For this review, take the finished solid that the model builds, in its own axes (mm). A direction names the side the tool comes from. Round coordinates to 2 decimals unless told otherwise and drop trailing zeros. Write each loop counter-clockwise with the first axis right and the second up, starting at its lowest first coordinate (ties: lowest second). Pieces come first, ordered by that corner, then holes. Notation, with made-up numbers: (65.25, -11.75) -> (88.25, -11.75) arc R24 cw to (88.25, 1.25) -> close; hole circle Ø7 at (3, -40). An arc over 180 degrees is marked (long way). Write item = value, one per line. Start each with the question number.
Autodesk Inventor part; units mm, degrees
ref_plane "Work Plane6" through (0, 0, 176.4284) normal (0, 0, 1) x (1, 0, 0)
ref_plane "Work Plane12" through (0, 0, 148.9464) normal (0, 0, 1) x (1, 0, 0)
ref_plane "Work Plane13" through (0, 0, 49.7586) normal (0, 0, -1) x (-1, 0, 0)
sketch "Sketch1" plane through (0, 0, 0) normal (0, 0, 1) x (1, 0, 0)
  circle A0 centre (0, 0) radius 4.7625
  line L0 (-1.5875, 6.35) -> (1.5875, 6.35)
  line L1 (1.5875, 6.35) -> (1.5875, 3.175)
  line L2 (1.5875, 3.175) -> (-1.5875, 3.175)
  line L3 (-1.5875, 3.175) -> (-1.5875, 6.35)
  dimension "d0" = 9.525
  dimension "d43" = 3.175
  dimension "d44" = 3.175
  dimension "d45" = 1.5875
  dimension "d46" = 6.35
extrude "Extrusion1" add sketch "Sketch1" along normal blind 165.05 contours A0 L3 L2 L1 | L1 L2 L3 A0
ref_plane "Work Plane6" through (0, 0, 176.4284) normal (0, 0, 1) x (1, 0, 0)
ref_plane "Work Plane12" through (0, 0, 148.9464) normal (0, 0, 1) x (1, 0, 0)
sketch "Sketch10" plane through (0, 0, 148.9464) normal (0, 0, 1) x (1, 0, 0)
  circle A0 centre (0, 0) radius 3.8481
  circle A1 centre (0, 0) radius 4.7625
extrude "Extrusion11" cut sketch "Sketch10" along normal blind 1.143
ref_plane "Work Plane13" through (0, 0, 49.7586) normal (0, 0, -1) x (-1, 0, 0)
sketch "Sketch11" plane through (0, 0, 49.7586) normal (0, 0, -1) x (-1, 0, 0)
  circle A0 centre (0, 0) radius 4.7625
  circle A1 centre (0, 0) radius 3.8481
  circle A2 centre (0, 0) radius 4.7625
extrude "Extrusion12" cut sketch "Sketch11" along normal blind 1.143
ref_plane "Work Plane14" through (0, 0, 26.797) normal (0, 0, -1) x (-1, 0, 0)
sketch "Sketch12" plane through (0, 0, 26.797) normal (0, 0, -1) x (-1, 0, 0)
  circle A0 centre (0, 0) radius 3.8481
  circle A1 centre (0, 0) radius 4.7625
extrude "Extrusion13" cut sketch "Sketch12" along normal blind 1.143
ref_plane "Work Plane15" through (0, 0, 148.921) normal (0, 0, 1) x (1, 0, 0)
extrude "Extrusion14" cut sketch "Sketch1" along normal through all contours L1 L2 L3 A0 | A0 L3 L0 L1 picked at (-0.1794, 3.694)
equation "\"d44\" = d43"
properties part number "vertical drive shaft"
1. Clearance check with flat-ended pins moving along their axes: pin 1 Ø1.5 at (x, z) = (2.5, 83) entering from -Y; pin 2 Ø1 at (x, y) = (1.5, -1) entering from -Z; pin 3 Ø0.7 at (y, z) = (4, 76.5) entering from +X; pin 4 Ø0.7 at (y, z) = (4, 57.5) entering from -X. State where each tip first meets the part, or that it passes through.
2. Consider section B-B, the plane z = 145.5. Give the boundary of the cut face in (x, y) (1 decimal).
3. Consider section C-C, the plane y = -2.5. Give the boundary of the cut face in (x, z).
4. Wall thickness on L1, parallel to Z at x = 0.25, y = -4.5; L2, parallel to X at y = 3.5, z = 20; L3, parallel to X at y = 0.5, z = 109: over which ranges is each line inside the solid? List them lowest first. Write a range as from..to.
5. Draft analysis for pull direction Z (two halves, no side actions). For faces 1 (the cylindrical face through (0.19, -4.76, 37.55)), 2 (the flat face through (0, -4, 26.797)), 3 (the flat face through (0, 0, 0)), 4 (the flat face through (0, 0, 165.05)), state which applies: +Z half, -Z half, draft (parallel to the pull), parting line (faces both ways), or undercut.
6. Machinability: for faces 5 (the cylindrical face through (0.19, -4.76, 12.65)), 6 (the cylindrical face through (-0.146, -3.845, 49.195)), 7 (the flat face through (0, 3.175, 81)), which of the approach directions +Z, -Z, +X, -X, +Y, -Y give a long, thin tool a straight path to every point of the face, cutting with its end or side? Answer none if there is none.
Outcome:
q1.pin_1 = -4.43
q1.pin_2 = 0
q1.pin_3 = 3.06
q1.pin_4 = -3.06
q2.outline = (-1.6, 3.2) -> (-1.6, 4.5) arc R4.8 ccw (long way) to (1.6, 4.5) -> (1.6, 3.2) -> close
q3.outline = (-4.05, 0) -> (4.05, 0) -> (4.05, 25.65) -> (2.93, 25.65) -> (2.93, 26.8) -> (4.05, 26.8) -> (4.05, 48.62) -> (2.93, 48.62) -> (2.93, 49.76) -> (4.05, 49.76) -> (4.05, 148.95) -> (2.93, 148.95) -> (2.93, 150.09) -> (4.05, 150.09) -> (4.05, 165.05) -> (-4.05, 165.05) -> (-4.05, 150.09) -> (-2.93, 150.09) -> (-2.93, 148.95) -> (-4.05, 148.95) -> (-4.05, 49.76) -> (-2.93, 49.76) -> (-2.93, 48.62) -> (-4.05, 48.62) -> (-4.05, 26.8) -> (-2.93, 26.8) -> (-2.93, 25.65) -> (-4.05, 25.65) -> close
q4.L1 = 0..25.65, 26.8..48.62, 49.76..148.95, 150.09..165.05
q4.L2 = -3.23..-1.59, 1.59..3.23
q4.L3 = -4.74..4.74
q5.face_1 = draft
q5.face_2 = undercut
q5.face_3 = -Z half
q5.face_4 = +Z half
q6.face_5 = +Z, -Z
q6.face_6 = none
q6.face_7 = +Z, -Z, +Y
